For this review, use the dimensioned drawing (mm, ordinates from the lowest corner) and the shaded views. A direction names the side the tool comes from. Round coordinates to 2 decimals unless told otherwise and drop trailing zeros. Order: outer loops, then holes, each group sorted by start corner. A loop starts at its lowest first (then second) coordinate and runs counter-clockwise, first axis right, second up. Notation, with made-up numbers: (32, 80) - (42, 80) arc R30 ccw to (42, 102) - close; hole circle Ø1 at (80.25, -16). An arc over 180 degrees is marked (long way). Write item = value, one per line.
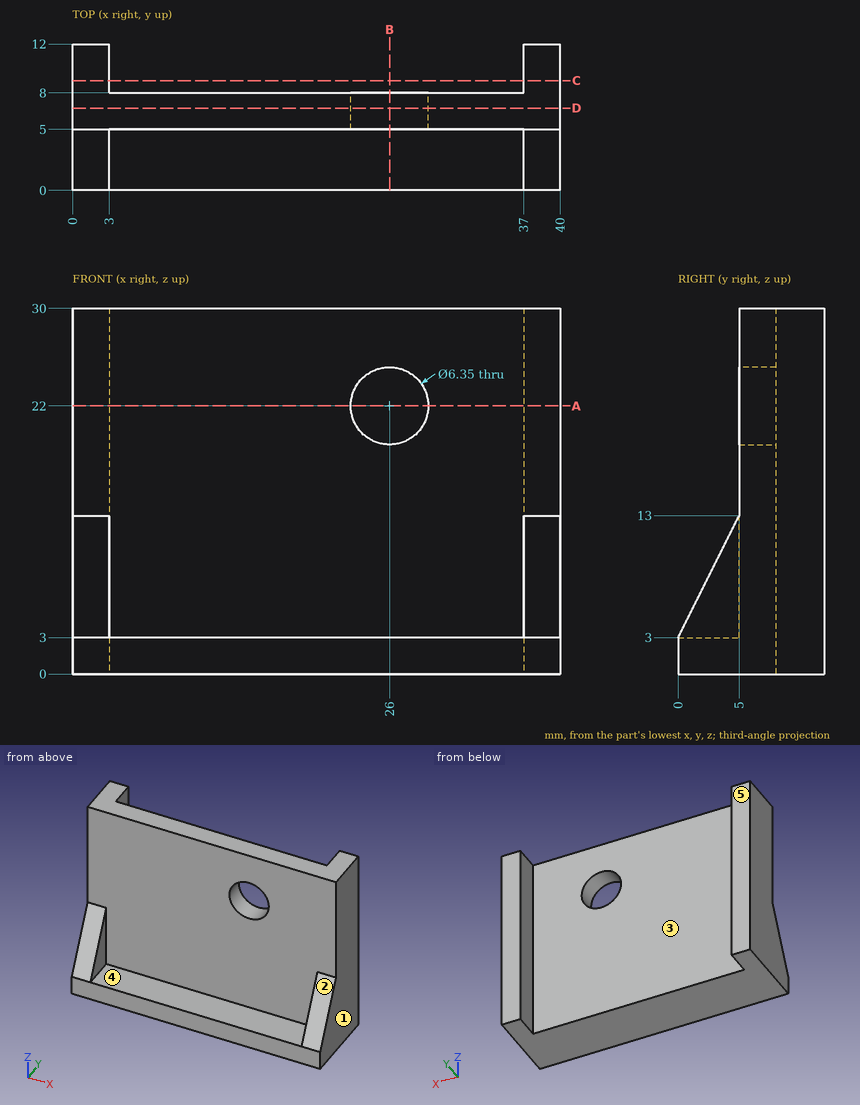
1) We need section B-B on x = 26. Write out the cut boundary in (y, z) (3 decimals), and give its area (4 significant figures).
Findings:
outline = (0, 0) - (8, 0) - (8, 18.825) - (5, 18.825) - (5, 3) - (0, 3) - close; (5, 25.175) - (8, 25.175) - (8, 30) - (5, 30) - close
area = 85.95 mm^2
2) We need section D-D on y = 6.75. Write out the cut boundary in (x, z) (3 decimals).
Findings:
outline = (0, 0) - (40, 0) - (40, 30) - (0, 30) - close; hole circle Ø6.35 at (26, 22)
3) For the marked faces 4 and 5, list the 3-axis set-ups (+Z, -Z, +X, -X, +Y, -Y) from which the entire face can be reached by the end or side of a thin tool; tool diameter is ignored.
Findings:
face_4 = +Z, -Y
face_5 = +Z, -Z, +X, -X, +Y
4) The part is to be moulded in two halves that separate along X. For the marked faces 1, 2 and 3, say which applies: released by +X, released by -X, zero draft, split by the parting line, or undercut.
Findings:
face_1 = released by +X
face_2 = zero draft
face_3 = undercut
5) Clearance check with flat-ended pins moving along their axes: pin 1 Ø3 at (x, z) = (10, 4.5) entering from +Y; pin 2 Ø2.5 at (x, y) = (15, 3) entering from +Z; pin 3 Ø1.5 at (x, z) = (13.5, 17.5) entering from -Y; pin 4 Ø4 at (x, z) = (26, 22) entering from +Y. State where each tip first meets the part, or that it passes through.
Findings:
pin_1 = 8
pin_2 = 3
pin_3 = 5
pin_4 = through
6) We need section C-C on y = 9. Write out the cut boundary in (x, z).
Findings:
outline = (0, 0) - (3, 0) - (3, 30) - (0, 30) - close; (37, 0) - (40, 0) - (40, 30) - (37, 30) - close
7) We need section A-A on z = 22. Write out the cut boundary in (x, y) (3 decimals), and give its area (3 significant figures).
Findings:
outline = (0, 5) - (22.825, 5) - (22.825, 8) - (3, 8) - (3, 12) - (0, 12) - close; (29.175, 5) - (40, 5) - (40, 12) - (37, 12) - (37, 8) - (29.175, 8) - close
area = 125 mm^2
8) To check wall thickness, follow L1, parallel to X at y = 10.5, z = 18.5; L2, parallel to X at y = 7, z = 22 (3 decimals); L3, parallel to Y at x = 34, z = 11.75. State the ranges of each line that lie inside material, in increasing order. Write a range as from..to.
Findings:
L1 = 0..3, 37..40
L2 = 0..22.825, 29.175..40
L3 = 5..8
